from build123d import *

# Parameters (mm, degrees)
F0_W      = 70
F0_H      = 3
F1_DEPTH  = 15
F2_R      = 1.65
F3_DEPTH  = 25
F4_R      = 2.75
F5_DEPTH  = 1
F6_R      = 1.65
F7_DEPTH  = 3
F8_R      = 1.65
F9_DEPTH  = 3
F8_R_2    = 2.75
F10_DEPTH = 1
F11_R     = 1.65
F12_DEPTH = 1


with BuildPart() as f1:
    # F0 (on Top) → F1 (new body)
    with BuildSketch(Plane.XY):
        Rectangle(F0_W, F0_H)
        Polygon((35, 16.5), (35, 1.5), (35, -1.5), (38, -1.5), (38, 16.5), align=None)
    extrude(amount=F1_DEPTH)

    # F2 (on face) → F3 (cut)
    with BuildSketch(Plane(origin=(35, 0, 0), x_dir=(0, -1, 0), z_dir=(-1, 0, 0))):
        with Locations((-9, 7.5)):
            Circle(F2_R)
    extrude(amount=-F3_DEPTH, mode=Mode.SUBTRACT)

    # F4 (on face) → F5 (cut)
    with BuildSketch(Plane.YZ.offset(38)):
        with Locations((9, 7.5)):
            Circle(F4_R)
    extrude(amount=-F5_DEPTH, mode=Mode.SUBTRACT)

    # F6 (on face) → F7 (cut, through all)
    with BuildSketch(Plane.XZ.offset(1.5)):
        with Locations((-20, 7.5)):
            Circle(F6_R)
    extrude(amount=-F7_DEPTH, mode=Mode.SUBTRACT)

    # F8 (on face) → F9 (cut, through all)
    with BuildSketch(Plane.XZ.offset(1.5)):
        with Locations((27.5, 7.5)):
            Circle(F8_R)
    extrude(amount=-F9_DEPTH, mode=Mode.SUBTRACT)

    # F8 (on face) → F10 (cut)
    with BuildSketch(Plane.XZ.offset(1.5)):
        with Locations((27.5, 7.5)):
            Circle(F8_R_2)
        with Locations((27.5, 7.5)):
            Circle(F8_R, mode=Mode.SUBTRACT)
    extrude(amount=-F10_DEPTH, mode=Mode.SUBTRACT)

    # F11 (on face) → F12 (cut)
    with BuildSketch(Plane(origin=(0, 1.5, 0), x_dir=(-1, 0, 0), z_dir=(0, 1, 0))):
        Polygon((21.674316, 10.4), (18.325684, 10.4), (16.651368, 7.5), (18.325684, 4.6), (21.674316, 4.6), (23.348632, 7.5), align=None)
        with Locations((20, 7.5)):
            Circle(F11_R, mode=Mode.SUBTRACT)
    extrude(amount=-F12_DEPTH, mode=Mode.SUBTRACT)


solid = f1.part
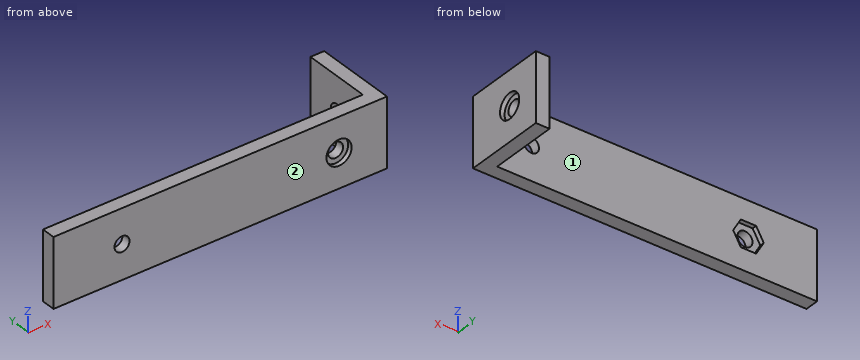
Input: part model. Units: mm. Frame: model coordinates. Face numbers are marked on the shaded views. A direction names the side the tool comes from. Give positions to 0.01 mm unless a question says otherwise; leave off trailing zeros. Order: outer loops, then holes, each group sorted by start corner. A loop starts at its lowest first (then second) coordinate and runs counter-clockwise, first axis right, second up.
Q1. Section D-D on x = 9.5. Output: boundary loops of the cut face in (y, z).
Checked values:
outline: (-1.5, 0) - (1.5, 0) - (1.5, 15) - (-1.5, 15) - close
Q2. Ray query, probe 1 along Z at (x, y) = (27.5, -1.3); probe 2 along Z at (x, y) = (-20, -0.15); probe 3 along Y at (x, z) = (28.5, 2.25). Return the intervals inside material, ascending.
Checked values:
probe 1: z = 0 to 4.75, 10.25 to 15
probe 2: z = 0 to 5.85, 9.15 to 15
probe 3: y = -1.5 to 1.5
Q3. Set-up query: the marked faces 1 and 2. Return all of +Z, -Z, +X, -X, +Y, -Y with unobstructed straight access to the full face (end or side cutting, diameter ignored); none if empty.
Checked values:
face 1: +Z, -Z, -X, +Y
face 2: +Z, -Z, +X, -X, -Y
Q4. Section A-A on x = -20. Output: boundary loops of the cut face in (y, z), and give its area (3 significant figures).
Checked values:
outline: (-1.5, 0) - (1.5, 0) - (1.5, 4.6) - (0.5, 4.6) - (0.5, 5.85) - (-1.5, 5.85) - close; (-1.5, 9.15) - (0.5, 9.15) - (0.5, 10.4) - (1.5, 10.4) - (1.5, 15) - (-1.5, 15) - close
area: 32.6 mm2
Q5. Section C-C on z = 11.5. Output: boundary loops of the cut face in (x, y).
Checked values:
outline: (-35, -1.5) - (38, -1.5) - (38, 16.5) - (35, 16.5) - (35, 1.5) - (-35, 1.5) - close
Q6. Section B-B on y = 9. Output: boundary loops of the cut face in (x, z), and give its area (3 significant figures).
Checked values:
outline: (35, 0) - (38, 0) - (38, 4.75) - (37, 4.75) - (37, 5.85) - (35, 5.85) - close; (35, 9.15) - (37, 9.15) - (37, 10.25) - (38, 10.25) - (38, 15) - (35, 15) - close
area: 32.9 mm2
Q7. Contact query for flat-ended pins moving along their axis: pin 1 Ø5.5 at (x, z) = (-20, 7.5) entering from -Y; pin 2 Ø7.5 at (y, z) = (5.5, 10.5) entering from -X; pin 3 Ø1.6 at (y, z) = (10.5, 7) entering from +X; pin 4 Ø6.5 at (x, z) = (-19, 7) entering from +Y. Output: stop coordinate, or through.
Checked values:
pin 1: stops at y = -1.5
pin 2: stops at x = 35
pin 3: stops at x = 37
pin 4: stops at y = 1.5
